Design review of the part built by this model. Coordinates are the model's own, in mm. A direction names the side the tool comes from. Coordinates: 2 decimals unless noted, no trailing zeros. Loops run counter-clockwise (first coordinate to the right, second up) from the corner with the lowest first, then second, coordinate; pieces in that order, holes last. Notation, with made-up numbers: (83, -28.75) -> (89, -28.75) arc R19 ccw to (89, -10.75) -> close; hole circle Ø5 at (80.5, 86). An arc over 180 degrees is marked (long way). Answer in a Markdown table with one row per item.
Autodesk Inventor part; units mm, degrees
ref_plane "YZ Plane" through (0, 0, 0) normal (1, 0, 0) x (0, 1, 0)
ref_plane "XZ Plane" through (0, 0, 0) normal (0, 1, 0) x (-1, 0, 0)
ref_plane "XY Plane" through (0, 0, 0) normal (0, 0, 1) x (1, 0, 0)
sketch "Sketch1" plane through (0, 0, 0) normal (0, 1, 0) x (-1, 0, 0)
  line L0 (13.5, 13.95) -> (2.5, 13.95)
  line L1 (0, 11.45) -> (0, -11.45)
  line L2 (16, -11.45) -> (16, 11.45)
  line L3 (3.15, -13.95) -> (3.15, -15.03)
  line L4 (3.15, -15.03) -> (12, -15.03)
  line L5 (12, -15.03) -> (12, -13.95)
  line L6 (2.5, -13.95) -> (3.15, -13.95)
  line L7 (12, -13.95) -> (13.5, -13.95)
  arc A0 (16, 11.45) -> (13.5, 13.95) centre (13.5, 11.45) ccw
  arc A1 (2.5, 13.95) -> (0, 11.45) centre (2.5, 11.45) ccw
  arc A2 (0, -11.45) -> (2.5, -13.95) centre (2.5, -11.45) ccw
  arc A3 (13.5, -13.95) -> (16, -11.45) centre (13.5, -11.45) ccw
  point P0 (0, 0)
  point P1 (0, 0)
  dimension "d1" = 16
  dimension "d3" = 8.85
  dimension "d4" = 4
  dimension "d5" = 27.9
  dimension "d6" = 2.5
  dimension "d7" = 1.08
extrude "Extrusion1" add sketch "Sketch1" along normal blind 10.3
sketch "Sketch2" plane through (0, 10.3, 0) normal (0, 1, 0) x (1, 0, 0)
  line L0 (-16, 11.45) -> (-16, -11.45)
  line L1 (-12, 13.95) -> (-13.5, 13.95)
  line L2 (0, -11.45) -> (0, 11.45)
  line L3 (-13.5, -13.95) -> (-2.5, -13.95)
  point P0 (0, 0)
  point P1 (-13.2, 11.15)
  point P2 (-2.8, -11.15)
  dimension "d10" = 2.8
  dimension "d11" = 2.8
  dimension "d12" = 2.8
  dimension "d13" = 2.8
  dimension "d48" = 22.3
  dimension "d49" = 10.4
hole "Hole1" at (-13.2, 10.3, -11.15) at (-2.8, 10.3, 11.15) direction (0, -1, 0) diameter 3.1 end through all
sketch "Sketch3" plane through (-16, 0, -11.45) normal (-1, 0, 0) x (0, 0, 1)
  line L0 (10.65, 2.9) -> (8.65, 2.9)
  line L1 (8.65, 2.9) -> (8.65, 7.4)
  line L2 (8.65, 7.4) -> (10.65, 7.4)
  line L3 (10.65, 7.4) -> (10.65, 2.9)
  line L4 (14.9, 2.9) -> (12.9, 2.9)
  line L5 (12.9, 2.9) -> (12.9, 7.4)
  line L6 (12.9, 7.4) -> (14.9, 7.4)
  line L7 (14.9, 7.4) -> (14.9, 2.9)
  line L8 (21.9, 2.9) -> (19.15, 2.9)
  line L9 (19.15, 2.9) -> (19.15, 7.4)
  line L10 (19.15, 7.4) -> (21.9, 7.4)
  line L11 (21.9, 7.4) -> (21.9, 2.9)
  line L12 (25.4, 0) -> (25.4, 10.3) construction
  line L13 (25.4, 5.15) -> (-3.58, 5.15) construction
  line L14 (-3.58, 0) -> (-3.58, 10.3) construction
  point P0 (11.45, 0)
  point P1 (21.9, 5.15)
  point P2 (10.91, 5.15)
  dimension "d21" = 3.5
  dimension "d22" = 2.75
  dimension "d23" = 4.25
  dimension "d24" = 2
  dimension "d25" = 2
  dimension "d26" = 2.25
  dimension "d27" = 4.5
extrude "Extrusion2" cut sketch "Sketch3" against normal blind 3.75
sketch "Sketch4" plane through (0, 10.3, 0) normal (0, 1, 0) x (1, 0, 0)
  line L0 (-16, -3.45) -> (-16, -1.45) construction
  line L1 (-16, -3.45) -> (-12.25, -3.45) construction
  line L2 (-12.25, -3.45) -> (-12.25, -1.45) construction
  line L3 (-16, -1.45) -> (-12.25, -1.45) construction
  line L4 (-16, 0.8) -> (-16, 2.8) construction
  line L5 (-16, 0.8) -> (-12.25, 0.8) construction
  line L6 (-12.25, 0.8) -> (-12.25, 2.8) construction
  line L7 (-16, 2.8) -> (-12.25, 2.8) construction
  line L8 (-14, -2.45) -> (-14, 1.7199) construction
  line L9 (-14, -2.45) -> (-12.25, -2.45) construction
  line L10 (-12.25, -3.45) -> (-12.25, -1.45) construction
  line L11 (-14, 1.7199) -> (-12.25, 1.7199) construction
  line L12 (-12.25, 0.8) -> (-12.25, 2.8) construction
  point P0 (0, 0)
  dimension "d30" = 2
hole "Hole2" at (-14, 10.3, 2.45) at (-14, 10.3, -1.7199) direction (0, -1, 0) diameter 0.75 end through all
sketch "Sketch5" plane through (-3.15, 0, -15.03) normal (0, 0, -1) x (-1, 0, 0)
  line L0 (1.6, 7.525) -> (1.1, 7.525)
  line L1 (1.1, 7.525) -> (1.1, 2.775)
  line L2 (1.1, 2.775) -> (1.6, 2.775)
  line L3 (1.6, 2.775) -> (1.6, 7.525)
  line L4 (12.85, 0) -> (12.85, 10.3) construction
  line L5 (12.85, 5.15) -> (1.6, 5.15) construction
  point P0 (-3.15, 0)
  dimension "d38" = 0.5
  dimension "d39" = 4.75
  dimension "d40" = 11.25
extrude "Extrusion3" cut sketch "Sketch5" against normal blind 0.25
sketch "Sketch6" plane through (0, 0, 11.45) normal (1, 0, 0) x (0, 0, -1)
  line L0 (12.5, 8.375) -> (13.35, 8.375)
  line L1 (13.35, 8.375) -> (13.35, 1.925)
  line L2 (13.35, 1.925) -> (12.5, 1.925)
  line L3 (12.5, 1.925) -> (12.5, 8.375)
  line L4 (-2.5, 0) -> (-2.5, 10.3)
  line L5 (-2.5, 0) -> (-2.5, 10.3)
  line L6 (-2.5, 5.15) -> (12.5, 5.15) construction
  point P0 (11.45, 0)
  dimension "d43" = 0.85
  dimension "d44" = 6.45
  dimension "d45" = 15
extrude "Extrusion4" cut sketch "Sketch6" against normal blind 0.25
properties part number "Housing" material "ABS Plastic"
(1) Take a section at A-A on x = -13.2. Give the boundary of the cut face in (y, z).
Evaluation:
| item | result |
|---|---|
| outline | (0, -13.95) -> (10.3, -13.95) -> (10.3, -12.7) -> (0, -12.7) -> close; (0, -9.6) -> (10.3, -9.6) -> (10.3, 13.95) -> (0, 13.95) -> close; hole (2.9, -2.8) -> (7.4, -2.8) -> (7.4, -0.8) -> (2.9, -0.8) -> close; hole (2.9, 1.45) -> (7.4, 1.45) -> (7.4, 3.45) -> (2.9, 3.45) -> close; hole (2.9, 7.7) -> (7.4, 7.7) -> (7.4, 10.45) -> (2.9, 10.45) -> close |
(2) To check wall thickness, follow probe 1 along Z at (x, y) = (-13.2, 2.75); probe 2 along Z at (x, y) = (-14, 2.3) (3 decimals); probe 3 along X at (y, z) = (7.75, -11.15). State the ranges of each line that lie inside material, in increasing order.
Evaluation:
| item | result |
|---|---|
| probe 1 | z = -13.95 to -12.7, -9.6 to 13.95 |
| probe 2 | z = -13.899 to -12.478, -9.822 to -2.095, -1.345 to 2.075, 2.825 to 13.899 |
| probe 3 | x = -16 to -14.75, -11.65 to 0 |
(3) For pin 1 (1 mm diameter, centred on y = 4.5, z = 2.5, fed in from -X); pin 2 (0.5 mm diameter, centred on y = 5, z = -14.5, fed in from -X); pin 3 (1.9 mm diameter, centred on x = -14, y = 5, fed in from -Z); pin 4 (3 mm diameter, centred on x = -2.8, z = 11.15, fed in from +Y), all flat-tipped, find the tip position at first contact; note any pin that passes through.
Evaluation:
| item | result |
|---|---|
| pin 1 | stops at x = -12.25 |
| pin 2 | stops at x = -12 |
| pin 3 | stops at z = -13.95 |
| pin 4 | passes through |
(4) Take a section at C-C on x = -2.8. Give the boundary of the cut face in (y, z), and give its area (3 significant figures).
Evaluation:
| item | result |
|---|---|
| outline | (0, -13.95) -> (10.3, -13.95) -> (10.3, 9.6) -> (0, 9.6) -> close; (0, 12.7) -> (10.3, 12.7) -> (10.3, 13.95) -> (0, 13.95) -> close |
| area | 255 mm² |
(5) Take a section at B-B on z = -11.15. Give the boundary of the cut face in (x, y).
Evaluation:
| item | result |
|---|---|
| outline | (-16, 0) -> (-14.75, 0) -> (-14.75, 10.3) -> (-16, 10.3) -> close; (-11.65, 0) -> (0, 0) -> (0, 10.3) -> (-11.65, 10.3) -> close |
(6) Tool access review of faces 1 (the flat face through (-12.25, 5, 2)), 2 (the cylindrical face through (-15.287, 5.078, -13.198)), 3 (the flat face through (-3.15, 5.1, -14.5)), 4 (the flat face through (-0.25, 5.2, -1.5)), 5 (the cylindrical face through (-11.687, 5.078, -11.486)): name each direction out of +Z, -Z, +X, -X, +Y, -Y from which nothing blocks a thin tool from reaching the whole face with its end or side.
Evaluation:
| item | result |
|---|---|
| face 1 | -X |
| face 2 | -Z, -X, +Y, -Y |
| face 3 | -Z, +X, +Y, -Y |
| face 4 | +X |
| face 5 | +Y, -Y |
(7) Take a section at D-D on y = 1. Give the boundary of the cut face in (x, z) (3 decimals).
Evaluation:
| item | result |
|---|---|
| outline | (-16, -11.45) arc R2.5 ccw to (-13.5, -13.95) -> (-12, -13.95) -> (-12, -15.03) -> (-3.15, -15.03) -> (-3.15, -13.95) -> (-2.5, -13.95) arc R2.5 ccw to (0, -11.45) -> (0, 11.45) arc R2.5 ccw to (-2.5, 13.95) -> (-13.5, 13.95) arc R2.5 ccw to (-16, 11.45) -> close; hole circle Ø3.1 at (-13.2, -11.15); hole circle Ø0.75 at (-14, -1.72); hole circle Ø0.75 at (-14, 2.45); hole circle Ø3.1 at (-2.8, 11.15) |
(8) Draft analysis for pull direction Z (two halves, no side actions). For faces 6 (the flat face through (-8, 5, 13.95)), 7 (the cylindrical face through (-0.752, 5.078, -13.237)), 8 (the flat face through (-12, 5.1, -14.5)), 9 (the flat face through (-14, 5, 10.45)), state which applies: pulls with the +Z half, pulls with the -Z half, needs draft (parallel to the pull), parting line crosses it, or undercut.
Evaluation:
| item | result |
|---|---|
| face 6 | pulls with the +Z half |
| face 7 | pulls with the -Z half |
| face 8 | needs draft |
| face 9 | undercut |
